Autodesk Inventor part; units mm, degrees
ref_plane "YZ Plane" through (0, 0, 0) normal (1, 0, 0) x (0, 1, 0)
ref_plane "XZ Plane" through (0, 0, 0) normal (0, 1, 0) x (-1, 0, 0)
ref_plane "XY Plane" through (0, 0, 0) normal (0, 0, 1) x (1, 0, 0)
sketch "Sketch1" plane through (0, 0, 0) normal (0, 1, 0) x (-1, 0, 0)
  line L0 (6, 5) -> (0, 5)
  line L1 (0, 5) -> (0, -5)
  line L2 (0, -5) -> (6, -5)
  line L3 (6, -5) -> (6, 5)
  line L4 (6, 5) -> (0, 0)
  line L5 (0, 0) -> (6, -5)
  line L6 (6, -5) -> (0, -10)
  line L7 (0, 18) -> (-2, 18)
  line L8 (-2, 18) -> (-2, -18)
  line L9 (-2, -18) -> (0, -18)
  line L10 (0, -18) -> (0, 18)
  line L11 (6, 5) -> (0, 10)
  point P0 (0, -10)
  point P1 (0, -5)
  point P2 (0, 5)
extrude "Extrusion1" add sketch "Sketch1" along normal blind 340 contours L4 L1 L0 | L0 L10 L11 | L1 L10 L9 L8 L7 | L6 L10 L2 | L2 L1 L5
chamfer "Chamfer1" distance 0.1 angle 45 2 edges at (-6, 170, -5) (-6, 170, 5)
chamfer "Chamfer2" distance 1 angle 45 1 edges at (0, 170, 0)
sketch "Sketch2" plane through (0, 340, 0) normal (0, 1, 0) x (1, 0, 0)
  line L0 (-4, 12) -> (0, 12)
  line L1 (0, 12) -> (0, 8)
  line L2 (0, 8) -> (-4, 8)
  line L3 (-4, 8) -> (-4, 12)
  line L4 (-4, -12) -> (0, -12)
  line L5 (0, -12) -> (0, -8)
  line L6 (0, -8) -> (-4, -8)
  line L7 (-4, -8) -> (-4, -12)
  point P0 (0, 0)
extrude "Extrusion2" cut sketch "Sketch2" against normal blind 1000
properties part number "RailDerzavka"
Could you check a few things on this model? Use its own coordinates, in mm. A direction names the side the tool comes from. Coordinates: 2 decimals unless noted, no trailing zeros. Loops run counter-clockwise (first coordinate to the right, second up) from the corner with the lowest first, then second, coordinate; pieces in that order, holes last. Notation, with made-up numbers: M -1,78 L 58,78 A23 ccw 58,113 Z; hole C 89.25,-19 d8. An arc over 180 degrees is marked long. Put each result on its own line as item: value. Start each with the question number.
(1) Suppose I cut it at B-B on y = 153. Please give me the cut outline in (x, z), then the cut area to 3 significant figures.
(2) Suppose I cut it at C-C on z = 14.5. Please give me the cut outline in (x, y), then the cut area to 3 significant figures.
(3) Suppose I cut it at A-A on x = -4.5. Please give me the cut outline in (y, z), then the cut area to 3 significant figures.
(4) Thinking about a two-plate mould opening in Z: for faces 4 (the face through (-3.31, 167.62, -2.76)), 5 (the face through (0, 340, 0)), which applies, pulls with the +Z half, pulls with the -Z half, needs draft (parallel to the pull), parting line crosses it, or undercut?
(5) I need wall thicknesses on line 1 (Z direction, x = -5, y = 256); line 2 (Z direction, x = -1.5, y = 296); line 3 (X direction, y = 79.5, z = -16). Which ranges of each line are inside material? Lowest first, please. Write a range as from..to.
(6) Will these pins go through, and if not, where does the flat tip stop? P1, Ø4, axis at y = 303.5, z = -11, coming from the -X side; P2, Ø0.6, axis at y = 178, z = 0, coming from the -X side; P3, Ø1.9, axis at x = -1, y = 138, coming from the +Z side.
(7) For faces 1 (the face through (-3.382, 167.62, 2.818)), 2 (the face through (0, 168, 13)), 3 (the face through (0, 172, -13)), which set-ups out of +Z, -Z, +X, -X, +Y, -Y let a thin tool reach every point of the face, with its end or its side?
Solutions:
1. outline: M -5.92,-5.06 L -2.4,-8 L 0,-8 L 0,-18 L 2,-18 L 2,18 L 0,18 L 0,8 L -2.4,8 L -5.92,5.06 L -5.92,4.94 L -0.77,0.64 L -0.77,-0.64 L -5.92,-4.94 Z
1. area: 128 mm2
2. outline: M 0,0 L 2,0 L 2,340 L 0,340 Z
2. area: 680 mm2
3. outline: M 0,-6.25 L 340,-6.25 L 340,-3.75 L 0,-3.75 Z; M 0,3.75 L 340,3.75 L 340,6.25 L 0,6.25 Z
3. area: 1,700 mm2
4. face 4: undercut
4. face 5: needs draft
5. line 1: z = -5.83..-4.17, 4.17..5.83
5. line 2: z = -8..-1.25, 1.25..8
5. line 3: x = 0..2
6. P1: stops at x = 0
6. P2: stops at x = -0.77
6. P3: stops at z = 8
7. face 1: -X, +Y, -Y
7. face 2: +Z, -X, +Y, -Y
7. face 3: -Z, -X, +Y, -Y
